from build123d import *

# Parameters (mm, degrees)
SKETCH1_W           = 52
SKETCH1_H           = 34
BOSS_EXTRUDE1_DEPTH = 5
SKETCH2_R           = 0.625
BOSS_EXTRUDE2_DEPTH = 5
FILLET1_R           = 4


with BuildPart() as part:
    # Sketch1 → Boss-Extrude1 (new, symmetric)
    with BuildSketch(Plane.XY):
        Rectangle(SKETCH1_W, SKETCH1_H)
    extrude(amount=BOSS_EXTRUDE1_DEPTH, both=True)

    # Sketch2 → Boss-Extrude2 (add)
    with BuildSketch(Plane.XZ.offset(17)):
        with Locations(Location((-25, 1, 0), (0, 0, 90))):
            Circle(SKETCH2_R)
        with Locations(Location((-25, -1, 0), (0, 0, 90))):
            Circle(SKETCH2_R)
    extrude(amount=BOSS_EXTRUDE2_DEPTH)

    # Fillet1
    # the kernel refuses this fillet: 4 mm, written as the material it takes off along each edge
    with BuildSketch(Plane(origin=(-26, 27, 5), x_dir=(0, 0, -1), z_dir=(0, -1, 0)), Plane(origin=(-26, 27, -5), x_dir=(1, 0, 0), z_dir=(0, -1, 0))) as fillet1_piece_1:
        with BuildLine():
            CenterArc((FILLET1_R, FILLET1_R), FILLET1_R, 180, 90)
            Line((0, FILLET1_R), (0, 0))
            Line((0, 0), (FILLET1_R, 0))
        make_face()
    extrude(amount=54, mode=Mode.SUBTRACT)
    with BuildSketch(Plane(origin=(-36, -17, 5), x_dir=(0, 0, -1), z_dir=(1, 0, 0))) as fillet1_piece_2_section:
        with BuildLine():
            CenterArc((FILLET1_R, FILLET1_R), FILLET1_R, 180, 90)
            Line((0, FILLET1_R), (0, 0))
            Line((0, 0), (FILLET1_R, 0))
        make_face()
    fillet1_piece_2 = extrude(amount=72, mode=Mode.PRIVATE)
    fillet1_piece_2 = fillet1_piece_2 - Plane(origin=(-25, -16.094238655, 1), x_dir=(0, 0, 1), z_dir=(0, 1, 0)) * Cylinder(0.625, 160, mode=Mode.PRIVATE)
    add(fillet1_piece_2, mode=Mode.SUBTRACT)
    with BuildSketch(Plane(origin=(-36, -17, -5), x_dir=(0, 0, 1), z_dir=(1, 0, 0))) as fillet1_piece_3_section:
        with BuildLine():
            CenterArc((FILLET1_R, -FILLET1_R), FILLET1_R, 90, 90)
            Line((0, -FILLET1_R), (0, 0))
            Line((0, 0), (FILLET1_R, 0))
        make_face()
    fillet1_piece_3 = extrude(amount=72, mode=Mode.PRIVATE)
    fillet1_piece_3 = fillet1_piece_3 - Plane(origin=(-25, -16.094238658, -1), x_dir=(0, 0, 1), z_dir=(0, 1, 0)) * Cylinder(0.625, 160, mode=Mode.PRIVATE)
    add(fillet1_piece_3, mode=Mode.SUBTRACT)
    with BuildSketch(Plane(origin=(36, 17, -5), x_dir=(0, -1, 0), z_dir=(-1, 0, 0))) as fillet1_piece_4:
        with BuildLine():
            CenterArc((FILLET1_R, FILLET1_R), FILLET1_R, 180, 90)
            Line((0, FILLET1_R), (0, 0))
            Line((0, 0), (FILLET1_R, 0))
        make_face()
    extrude(amount=72, mode=Mode.SUBTRACT)
    with BuildSketch(Plane(origin=(36, 17, 5), x_dir=(0, -1, 0), z_dir=(-1, 0, 0))) as fillet1_piece_5:
        with BuildLine():
            CenterArc((FILLET1_R, -FILLET1_R), FILLET1_R, 90, 90)
            Line((0, -FILLET1_R), (0, 0))
            Line((0, 0), (FILLET1_R, 0))
        make_face()
    extrude(amount=72, mode=Mode.SUBTRACT)


solid = part.part
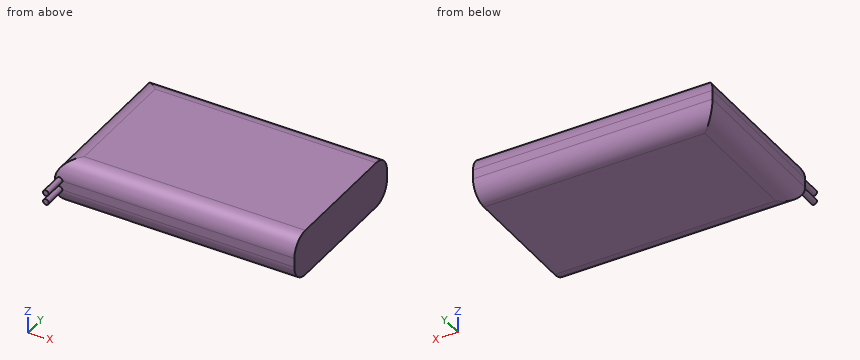
Here's how the part is built. I have some questions about the finished solid (model axes, mm). Round coordinates to 2 decimals unless told otherwise and drop trailing zeros. Order: outer loops, then holes, each group sorted by start corner. A loop starts at its lowest first (then second) coordinate and runs counter-clockwise, first axis right, second up. Notation, with made-up numbers: M -20.75,-20.75 L -0.75,-20.75 A20 cw -0.75,0.25 Z; hole C -29,58.5 d11. An arc over 180 degrees is marked long. Return JSON: item names as keys, results as strings. Group by question number.
1. If we section it at C-C on z = -3: List the corners of the cut face in (x, y) for me, then the cut area to 3 significant figures.
2. Please list where these lines run through material, in increasing order: probe 1 along X at (y, z) = (-16, 1.25); probe 2 along Y at (x, z) = (7.5, 0.75); probe 3 along Y at (x, z) = (-4.5, 2.25).
3. I'm going to push a flat-ended pin straight in: pin 1 Ø2 at (x, z) = (16, 0.5) entering from -Y. Where does the tip first touch, or does it pass through?
4. If we section it at A-A on x = 7.5: List the corners of the cut face in (y, z) for me.
5. If we section it at B-B on z = 4.25: List the corners of the cut face in (x, y) for me.
Reply:
{
 "1": {"outline": "M -25.46,-16.46 L 26,-16.46 L 26,16.46 L -25.46,16.46 Z", "area": "1,690 mm^2"},
 "2": {"probe 1": "-25.99 to 26", "probe 2": "-17 to 17", "probe 3": "-16.8 to 16.8"},
 "3": {"pin 1": "y = -17"},
 "4": {"outline": "M -17,-1 A4 ccw -13,-5 L 13,-5 A4 ccw 17,-1 L 17,1 A4 ccw 13,5 L -13,5 A4 ccw -17,1 Z"},
 "5": {"outline": "M -24.33,-15.33 L 26,-15.33 L 26,15.33 L -24.33,15.33 Z"}
}
